Can you work these out from the drawing? Everything is in mm from the part's minimum corner. A direction names the side the tool comes from. Give positions to 0.01 mm unless a question says otherwise; leave off trailing zeros. Order: outer loops, then holes, each group sorted by start corner. A loop starts at its lowest first (then second) coordinate and runs counter-clockwise, first axis right, second up. Notation, with made-up numbers: (52, -15.75) -> (68, -15.75) arc R25 ccw to (68, 9.25) -> close; hole circle Ø8 at (-31.5, 49). An arc over 180 degrees is marked (long way). Answer as CSV lines item,"result". Start each with the question number.
(1) I need wall thicknesses on L1, parallel to X at y = 112, z = 1.5 (3 decimals); L2, parallel to X at y = 101, z = 30; L3, parallel to Z at x = 22.5, y = 108.5 (3 decimals). Which ranges of each line are inside material? Lowest first, please.
(2) Will these pins go through, and if not, where does the flat tip stop? pin 1 Ø1 at (x, y) = (50, 88.5) entering from -Z (3 decimals); pin 2 Ø0.9 at (y, z) = (20.5, 30.5) entering from +X (3 decimals); pin 3 Ø10 at (x, z) = (11, 7) entering from +Y; pin 4 Ø1 at (x, z) = (75.5, 13.5) entering from -Y.
(3) I want a section at D-D (y = 35). Please give me the cut outline in (x, z) (3 decimals), plus the area to 3 significant figures.
(4) I want a section at B-B (z = 4). Please give me the cut outline in (x, y) (3 decimals).
(5) I want a section at C-C (y = 101.6). Please give me the cut outline in (x, z) (3 decimals), plus the area to 3 significant figures.
(6) I want a section at A-A (x = 38.1). Please give me the cut outline in (y, z) (3 decimals), plus the area to 3 significant figures.
(7) We'd pull the mould along X, two halves only. Please class the marked faces 3, 4 and 5: released by +X, released by -X, zero draft, split by the parting line, or undercut.
(8) On a 3-axis mill with a long thin cutter (end or side, diameter ignored), from which of +Z, -Z, +X, -X, +Y, -Y can I reach the whole of each face in a straight line? I mean the marked faces 1 and 2. Say none if no direction works.
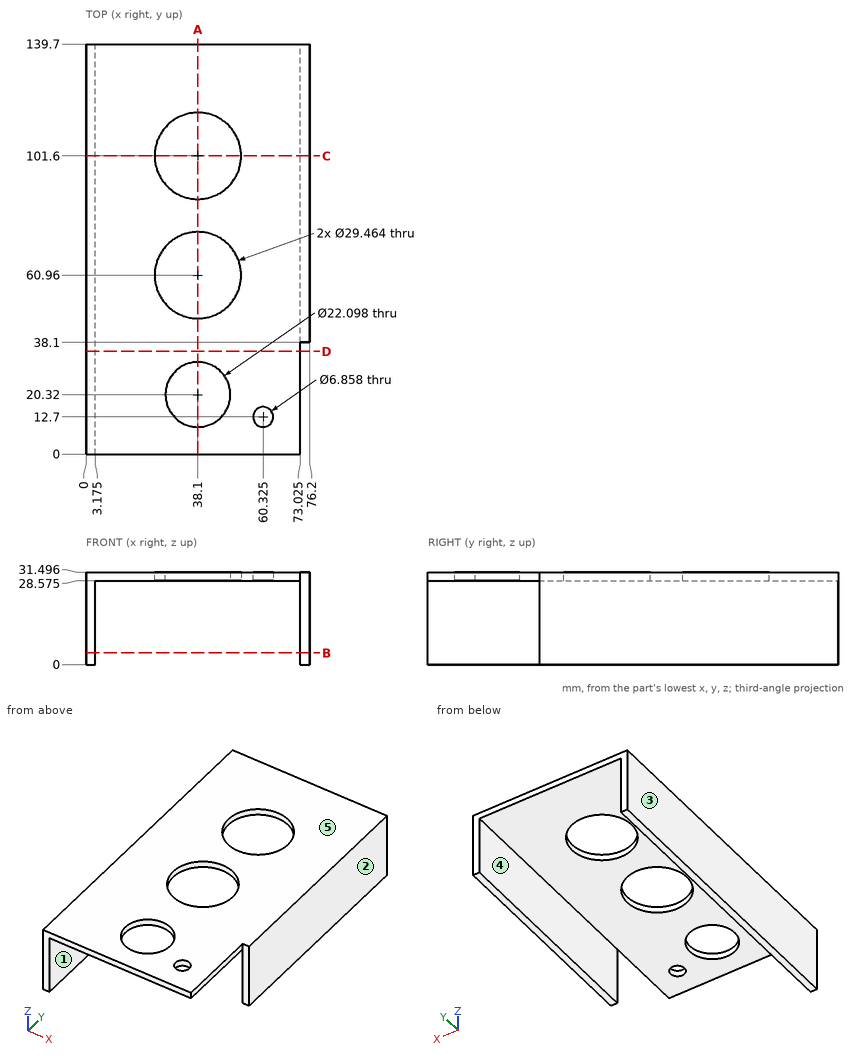
Final values:
1,L1,"0 to 3.175, 73.025 to 76.2"
1,L2,"0 to 23.38, 52.82 to 76.2"
1,L3,"28.575 to 31.496"
2,pin 1,"z = 28.575"
2,pin 2,"x = 73.025"
2,pin 3,"through"
2,pin 4,"y = 38.1"
3,outline,"(0, 0) -> (3.175, 0) -> (3.175, 28.575) -> (73.025, 28.575) -> (73.025, 31.496) -> (0, 31.496) -> close"
3,area,"304 mm²"
4,outline,"(0, 0) -> (3.175, 0) -> (3.175, 139.7) -> (0, 139.7) -> close; (73.025, 38.1) -> (76.2, 38.1) -> (76.2, 139.7) -> (73.025, 139.7) -> close"
5,outline,"(0, 0) -> (3.175, 0) -> (3.175, 28.575) -> (23.368, 28.575) -> (23.368, 31.496) -> (0, 31.496) -> close; (52.832, 28.575) -> (73.025, 28.575) -> (73.025, 0) -> (76.2, 0) -> (76.2, 31.496) -> (52.832, 31.496) -> close"
5,area,"318 mm²"
6,outline,"(0, 28.575) -> (9.271, 28.575) -> (9.271, 31.496) -> (0, 31.496) -> close; (31.369, 28.575) -> (46.228, 28.575) -> (46.228, 31.496) -> (31.369, 31.496) -> close; (75.692, 28.575) -> (86.868, 28.575) -> (86.868, 31.496) -> (75.692, 31.496) -> close; (116.332, 28.575) -> (139.7, 28.575) -> (139.7, 31.496) -> (116.332, 31.496) -> close"
6,area,"171 mm²"
7,face 3,"released by -X"
7,face 4,"undercut"
7,face 5,"zero draft"
8,face 1,"-Z, +Y, -Y"
8,face 2,"+Z, -Z, +X, +Y, -Y"
